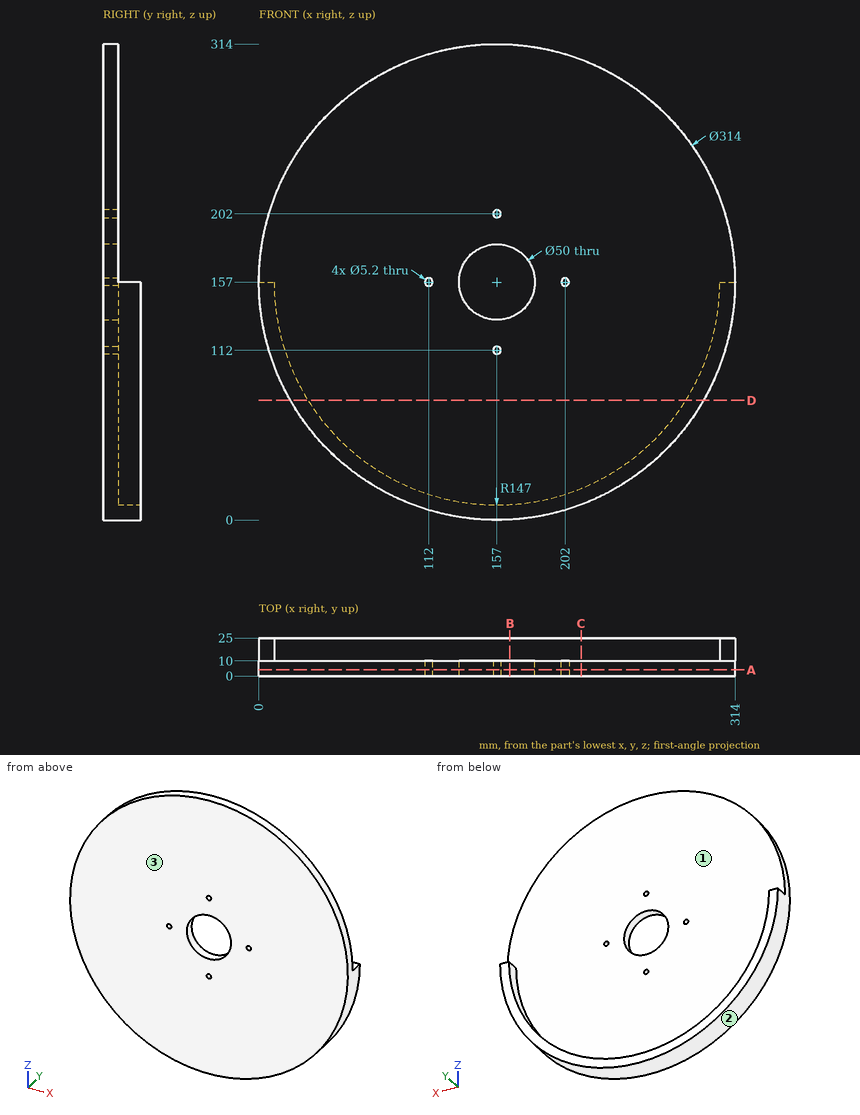
Geometry: see drawing. Coordinates: mm, zero at the bounding-box minimum. Round coordinates to 2 decimals unless told otherwise and drop trailing zeros. Order: outer loops, then holes, each group sorted by start corner. A loop starts at its lowest first (then second) coordinate and runs counter-clockwise, first axis right, second up. Notation, with made-up numbers: (-25, 8.5) -> (-18, 8.5) arc R22 ccw to (-18, 28.5) -> close; hole circle Ø1 at (17.25, -3). An arc over 180 degrees is marked (long way). Use CSV: the item, a comma, the result in double quotes.
(1) Section A-A on y = 4. Return the cut outline in (x, z), and give its area (3 significant figures).
Report:
outline,"circle Ø314 at (157, 157); hole circle Ø5.2 at (112, 157); hole circle Ø50 at (157, 157); hole circle Ø5.2 at (157, 112); hole circle Ø5.2 at (157, 202); hole circle Ø5.2 at (202, 157)"
area,"75,400 mm^2"
(2) Section B-B on x = 165.5. Return the cut outline in (y, z), and give its area (3 significant figures).
Report:
outline,"(0, 0.23) -> (25, 0.23) -> (25, 10.25) -> (10, 10.25) -> (10, 133.49) -> (0, 133.49) -> close; (0, 180.51) -> (10, 180.51) -> (10, 313.77) -> (0, 313.77) -> close"
area,"2,820 mm^2"
(3) Section C-C on x = 212.5. Return the cut outline in (y, z).
Report:
outline,"(0, 10.14) -> (25, 10.14) -> (25, 20.88) -> (10, 20.88) -> (10, 303.86) -> (0, 303.86) -> close"
(4) Ray query, L1, parallel to X at y = 5, z = 157; L2, parallel to Z at x = 157.5, y = 1.5 (3 decimals); L3, parallel to Y at x = 263, z = 63. Return the intervals inside material, ascending.
Report:
L1,"0 to 109.4, 114.6 to 132, 182 to 199.4, 204.6 to 314"
L2,"0.001 to 109.449, 114.551 to 132.005, 181.995 to 199.449, 204.551 to 313.999"
L3,"0 to 10"
(5) Pull-direction query (X, two-part tool) for the marked faces 1, 2 and 3; classes: +X half, -X half, draft (parallel to the pull), parting line (faces both ways), or undercut.
Report:
face 1,"undercut"
face 2,"parting line"
face 3,"draft"
(6) First-contact query: pin 1 Ø2 at (y, z) = (5, 63) entering from +X; pin 2 Ø8 at (x, y) = (72, 8.5) entering from -Z; pin 3 Ø5 at (x, y) = (310, 19) entering from +Z; pin 4 Ø4.5 at (x, z) = (112, 157) entering from +Y. Flat tips, straight axial feed; report the tip coordinate or a pass-through.
Report:
pin 1,"x = 283.49"
pin 2,"z = 22.51"
pin 3,"z = 157"
pin 4,"through"
(7) Section D-D on z = 79. Return the cut outline in (x, y), and give its area (3 significant figures).
Report:
outline,"(20.75, 0) -> (293.25, 0) -> (293.25, 25) -> (281.6, 25) -> (281.6, 10) -> (32.4, 10) -> (32.4, 25) -> (20.75, 25) -> close"
area,"3,070 mm^2"
